Job drawing, mm, ordinate dimensions from the low corner. One solid piece. A direction names the side the tool comes from. Give positions to 0.01 mm unless a question says otherwise; leave off trailing zeros. Order: outer loops, then holes, each group sorted by start corner. A loop starts at its lowest first (then second) coordinate and runs counter-clockwise, first axis right, second up. Notation, with made-up numbers: M 39.5,-1 L 98.5,-1 A21 cw 98.5,21 Z; hole C 63,-36 d5. An arc over 180 degrees is marked long. Put each result on its own line as item: value. Start each with the question number.
1) Cut at C-C (z = 0.7). Write the cut outline in (x, y), and give its area (3 significant figures).
2) Cut at D-D (x = 8.75). Write the cut outline in (y, z).
3) Two-plate mould, pull along X, no slides. Class the marked faces 4, 5 and 6: released by +X, released by -X, zero draft, split by the parting line, or undercut.
4) Cut at B-B (y = 3). Write the cut outline in (x, z), and give its area (3 significant figures).
5) Drill centre lines: line 1 (Y direction, x = 8.75, z = 0.2); line 2 (Y direction, x = 5.75, z = 0.65); line 3 (X direction, y = 7.25, z = 0.55). Where is each one in solid material? Low to high. Write a range as [from, to].
6) Pin check, flat tip, straight feed: pin 1 (1 mm diameter, centred on x = 4, y = 4, fed in from -Z). Stop position of the tip, or through.
7) Cut at A-A (x = 6). Write the cut outline in (y, z).
8) Tool access for the marked faces 1, 2 and 3: list every direction of +Z, -Z, +X, -X, +Y, -Y with a clear straight run to the whole face (end or side of a thin tool).
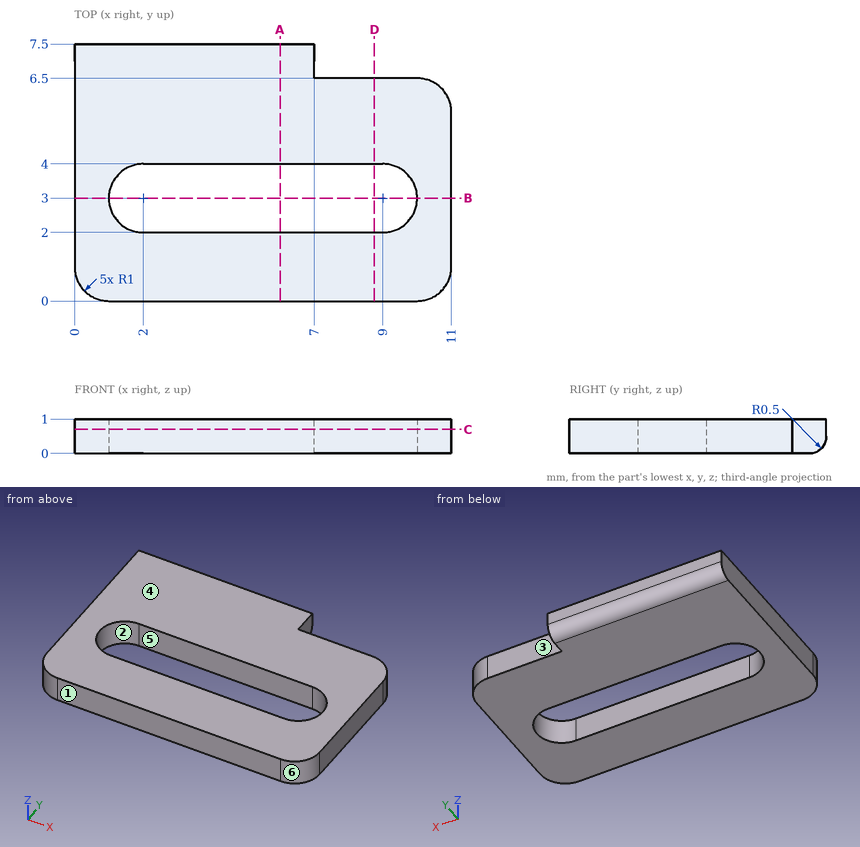
Solution:
1. outline: M 0,1 A1 ccw 1,0 L 10,0 A1 ccw 11,1 L 11,5.5 A1 ccw 10,6.5 L 7,6.5 L 7,7.5 L 0,7.5 Z; hole M 2,2 L 9,2 A1 ccw 9,4 L 2,4 A1 ccw Z
1. area: 60.7 mm²
2. outline: M 0,0 L 2,0 L 2,1 L 0,1 Z; M 4,0 L 6.5,0 L 6.5,1 L 4,1 Z
3. face 4: zero draft
3. face 5: undercut
3. face 6: released by +X
4. outline: M 0,0 L 1,0 L 1,1 L 0,1 Z; M 10,0 L 11,0 L 11,1 L 10,1 Z
4. area: 2.00 mm²
5. line 1: [0, 2], [4, 6.5]
5. line 2: [0, 2], [4, 7.5]
5. line 3: [0, 7]
6. pin 1: z = 0
7. outline: M 0,0 L 2,0 L 2,1 L 0,1 Z; M 4,0 L 7,0 A0.5 ccw 7.5,0.5 L 7.5,1 L 4,1 Z
8. face 1: +Z, -Z, +X, -X, -Y
8. face 2: +Z, -Z
8. face 3: +Z, -Z, +X, +Y
